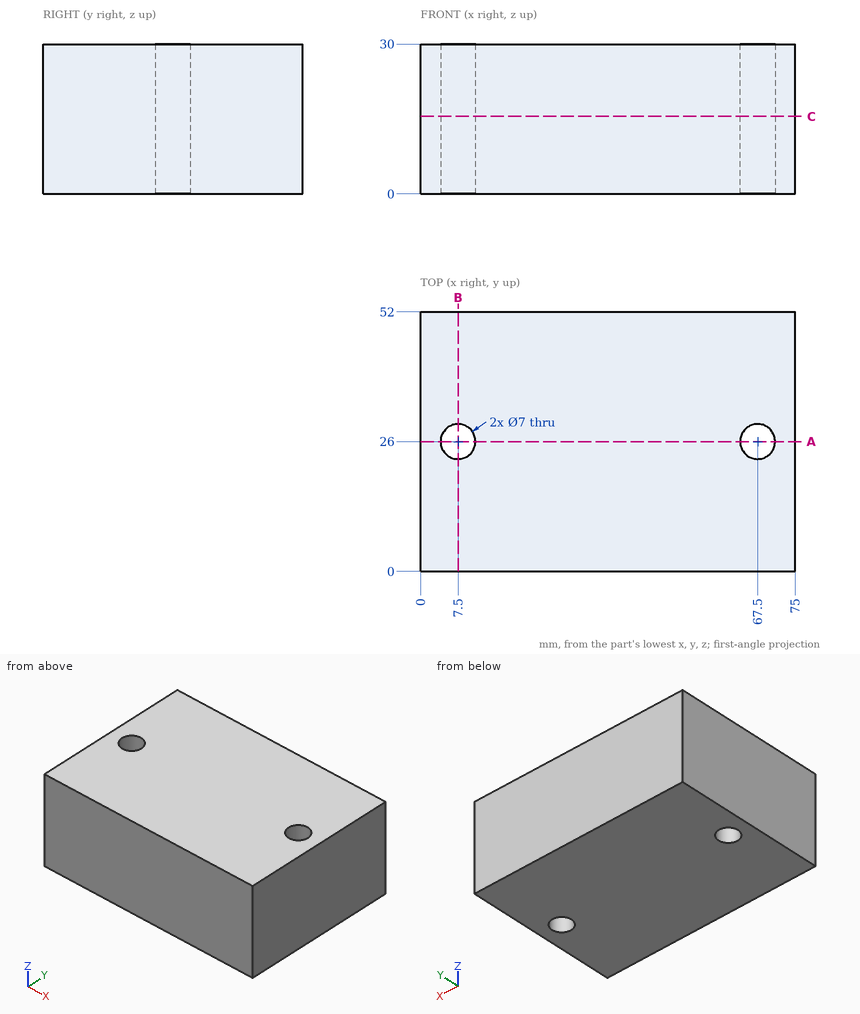
Could you check a few things on this drawing? It's one solid part, dimensions in mm from its lowest x, y, z. Give positions to 0.01 mm unless a question says otherwise; leave off trailing zeros. Write each loop counter-clockwise with the first axis right and the second up, starting at its lowest first coordinate (ties: lowest second). Pieces come first, ordered by that corner, then holes. Notation, with made-up numbers: (23.5, 34.25) -> (76.5, 34.25) arc R19 ccw to (76.5, 57.25) -> close; hole circle Ø4 at (27.5, 73). An arc over 180 degrees is marked (long way). Answer as CSV lines item,"result". Start each with the question number.
(1) I'm going to push a flat-ended pin straight in: pin 1 Ø9 at (x, y) = (67.5, 26) entering from -Z. Where does the tip first touch, or does it pass through?
(2) If we section it at C-C, the plane z = 15.5: Write out the boundary of the cut face in (x, y), and give its area (3 significant figures).
(3) Please list where these lines run through material, in increasing order: line 1 (Y direction, x = 67.5, z = 21.25); line 2 (X direction, y = 29, z = 24); line 3 (X direction, y = 26.5, z = 9.25).
(4) If we section it at B-B, the plane x = 7.5: Write out the boundary of the cut face in (y, z).
(5) If we section it at A-A, the plane y = 26: Write out the boundary of the cut face in (x, z).
Answer list:
1,pin 1,"z = 0"
2,outline,"(0, 0) -> (75, 0) -> (75, 52) -> (0, 52) -> close; hole circle Ø7 at (7.5, 26); hole circle Ø7 at (67.5, 26)"
2,area,"3,820 mm^2"
3,line 1,"0 to 22.5, 29.5 to 52"
3,line 2,"0 to 5.7, 9.3 to 65.7, 69.3 to 75"
3,line 3,"0 to 4.04, 10.96 to 64.04, 70.96 to 75"
4,outline,"(0, 0) -> (22.5, 0) -> (22.5, 30) -> (0, 30) -> close; (29.5, 0) -> (52, 0) -> (52, 30) -> (29.5, 30) -> close"
5,outline,"(0, 0) -> (4, 0) -> (4, 30) -> (0, 30) -> close; (11, 0) -> (64, 0) -> (64, 30) -> (11, 30) -> close; (71, 0) -> (75, 0) -> (75, 30) -> (71, 30) -> close"
